Check sheet for the modelled part. Datum: model origin and axes. Units: mm. A direction names the side the tool comes from. Give positions to 0.01 mm unless a question says otherwise; leave off trailing zeros. Order: outer loops, then holes, each group sorted by start corner. A loop starts at its lowest first (then second) coordinate and runs counter-clockwise, first axis right, second up.
Item 1: Sectioned sample at C-C on y = 1.5. Record the boundary of the cut face in (x, z).
Item 2: Sectioned sample at B-B on x = 0. Record the boundary of the cut face in (y, z).
Item 3: Sectioned sample at A-A on z = 0. Record the boundary of the cut face in (x, y).
Item 4: Gauge pin test, flat ends, axial feed: P1, Ø3, axis at y = 19, z = 3, coming from the +X side; P2, Ø4, axis at y = 12.5, z = 2, coming from the -X side; P3, Ø12, axis at y = 11, z = 4, coming from the +X side. Record the tip position at first contact, or that the pin passes through.
Item 5: Release check for a two-part mould opening along Y. For faces 1 (the flat face through (5, 8, -1)), 2 (the cylindrical face through (5.19, 12.93, -2.7)), 3 (the flat face through (0, 5, 0)), 4 (the flat face through (5, 7, -1)) record: released by +Y, released by -Y, zero draft, split by the parting line, or undercut.
Item 6: Access from +Z, -Z, +X, -X, +Y, -Y to the whole of each face (thin tool, end or side, straight path). Record for faces 5 (the cylindrical face through (1.457, 7.493, -4.626)), 6 (the flat face through (1.2, 0, -1.2)), 7 (the cylindrical face through (0.45, 2.46, -1.43)).
Item 7: Sectioned sample at D-D on y = 19.5. Record the boundary of the cut face in (x, z).
Item 8: Material ranges on line 1 along X through (y, z) = (3.7, 0); line 2 along Y through (x, z) = (-5, 11.5); line 3 along X through (y, z) = (1.5, -1), recorded low to high.
from build123d import *

# Parameters (mm, degrees)
SKETCH1_R           = 5.85
BOSS_EXTRUDE1_DEPTH = 21
SKETCH2_R           = 17.316392141
BOSS_EXTRUDE2_DEPTH = 2
CUT_EXTRUDE1_START  = 1
SKETCH3_R           = 5.85
SKETCH3_R_2         = 4.85
CUT_EXTRUDE1_DEPTH  = 1
SKETCH4_R           = 1.5
CUT_EXTRUDE2_DEPTH  = 5
BOSS_EXTRUDE4_START = 3
SKETCH5_R           = 8.85
SKETCH5_R_2         = 5.85
BOSS_EXTRUDE4_DEPTH = 3


with BuildPart() as part:
    # Sketch1 → Boss-Extrude1 (new body)
    with BuildSketch(Plane(origin=(0, 0, 0), x_dir=(1, 0, 0), z_dir=(0, 1, 0))):
        with Locations(Location((0, 0, 0), (0, 0, 90))):
            Circle(SKETCH1_R)
    extrude(amount=BOSS_EXTRUDE1_DEPTH)

    # Sketch2 → Boss-Extrude2 (add)
    with BuildSketch(Plane(origin=(0, 21, 0), x_dir=(1, 0, 0), z_dir=(0, 1, 0))):
        with Locations(Location((0, 0, 0), (0, 0, 270))):
            Circle(SKETCH2_R)
    extrude(amount=BOSS_EXTRUDE2_DEPTH)

    # Sketch3 → Cut-Extrude1 (cut)
    with BuildSketch(Plane(origin=(0, 8, 0), x_dir=(-1, 0, 0), z_dir=(0, -1, 0)).offset(CUT_EXTRUDE1_START)):
        with Locations(Location((0, 0, 0), (0, 0, 90))):
            Circle(SKETCH3_R)
        with Locations(Location((0, 0, 0), (0, 0, 90))):
            Circle(SKETCH3_R_2, mode=Mode.SUBTRACT)
    extrude(amount=-CUT_EXTRUDE1_DEPTH, mode=Mode.SUBTRACT)

    # Sketch4 → Cut-Extrude2 (cut)
    with BuildSketch(Plane.XZ):
        with Locations(Location((0, 0, 0), (0, 0, 270))):
            Circle(SKETCH4_R)
    extrude(amount=-CUT_EXTRUDE2_DEPTH, mode=Mode.SUBTRACT)

    # Sketch5 → Boss-Extrude4 (add)
    with BuildSketch(Plane.XZ.offset(-21).offset(BOSS_EXTRUDE4_START)):
        with Locations(Location((0, 0, 0), (0, 0, 90))):
            Circle(SKETCH5_R)
        with Locations(Location((0, 0, 0), (0, 0, 270))):
            Circle(SKETCH5_R_2, mode=Mode.SUBTRACT)
    extrude(amount=-BOSS_EXTRUDE4_DEPTH)


solid = part.part
Report:
1. outline: circle Ø11.7 at (0, 0); hole circle Ø3 at (0, 0)
2. outline: (0, -5.85) - (7, -5.85) - (7, -4.85) - (8, -4.85) - (8, -5.85) - (18, -5.85) - (18, -8.85) - (21, -8.85) - (21, -17.32) - (23, -17.32) - (23, 17.32) - (21, 17.32) - (21, 8.85) - (18, 8.85) - (18, 5.85) - (8, 5.85) - (8, 4.85) - (7, 4.85) - (7, 5.85) - (0, 5.85) - (0, 1.5) - (5, 1.5) - (5, -1.5) - (0, -1.5) - close
3. outline: (-17.32, 21) - (-8.85, 21) - (-8.85, 18) - (-5.85, 18) - (-5.85, 8) - (-4.85, 8) - (-4.85, 7) - (-5.85, 7) - (-5.85, 0) - (-1.5, 0) - (-1.5, 5) - (1.5, 5) - (1.5, 0) - (5.85, 0) - (5.85, 7) - (4.85, 7) - (4.85, 8) - (5.85, 8) - (5.85, 18) - (8.85, 18) - (8.85, 21) - (17.32, 21) - (17.32, 23) - (-17.32, 23) - close
4. P1: stops at x = 8.72
4. P2: stops at x = -5.85
4. P3: stops at x = 5.85
5. face 1: undercut
5. face 2: zero draft
5. face 3: released by -Y
5. face 4: undercut
6. face 5: none
6. face 6: +Z, -Z, +X, -X, -Y
6. face 7: -Y
7. outline: circle Ø17.7 at (0, 0)
8. line 1: x = -5.85 to -1.5, 1.5 to 5.85
8. line 2: y = 21 to 23
8. line 3: x = -5.76 to -1.12, 1.12 to 5.76
